Read the model definition and answer for the solid it produces. Units are mm, in the model's axes. Face numbers are marked on the shaded views. Coordinates: 2 decimals unless noted, no trailing zeros. Loops run counter-clockwise (first coordinate to the right, second up) from the corner with the lowest first, then second, coordinate; pieces in that order, holes last. Notation, with made-up numbers: (0, 72) - (11, 72) arc R22 cw to (11, 111) - close; hole circle Ø1 at (-30.5, 40.5). An arc over 180 degrees is marked (long way). Use CSV: the item, a comma, the result in double quotes.
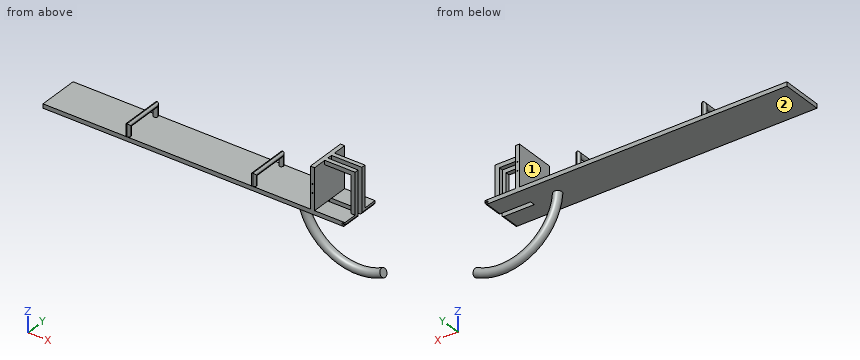
```python
from build123d import *

# Parameters (mm, degrees)
F1_DEPTH  = 20
F2_R      = 10
F5_R      = 20
F9_DEPTH  = 196.2
F11_R     = 2.5
F12_DEPTH = 30
F14_R     = 2.5
F15_DEPTH = 30
F18_DEPTH = 20
F21_DEPTH = 20
F23_DEPTH = 20
F26_DEPTH = 20


with BuildPart() as f1:
    # F0 (on Top) → F1 (new body)
    with BuildSketch(Plane.XY):
        Polygon((0, -98.1), (0, -12), (-155, -12), (-155, 0), (-155, 12), (0, 12), (0, 98.1), (-1441.76, 98.1), (-1441.76, -98.1), align=None)
    extrude(amount=-F1_DEPTH)

    # F2
    f2_edges = [f1.edges().sort_by_distance(p)[0] for p in [
        (0, -55.05, -20),
        (0, 55.05, -20),
    ]]
    fillet(f2_edges, radius=F2_R)

    # F6: sweep along a path in F4
    with BuildLine(Plane.XZ) as f6_path:
        ThreePointArc((-276.33, 0), (-148.7703707389, -227.3201555186), (111.7183092779, -236.8888390924))
    # F5 (on Top) → F6 (sweep)
    with BuildSketch(Plane.XY):
        with Locations((-276.33, 0)):
            Circle(F5_R)
    sweep(path=f6_path.line)

    # F8 (on offset) → F9 (join)
    with BuildSketch(Plane.XZ.offset(98.1)):
        Polygon((-155, 0), (-145, 0), (-145, 196.2), (-155, 196.2), (-165, 196.2), (-165, 0), align=None)
    extrude(amount=-F9_DEPTH)

    # F11 (on offset) → F12 (cut)
    with BuildSketch(Plane.XZ.offset(98.1)):
        with Locations((-155, 118.6)):
            Circle(F11_R)
        with Locations((-155, 77.6)):
            Circle(F11_R)
    extrude(amount=-F12_DEPTH, mode=Mode.SUBTRACT)

    # F14 (on offset) → F15 (cut)
    with BuildSketch(Plane(origin=(0, 98.1, 0), x_dir=(-1, 0, 0), z_dir=(0, 1, 0))):
        with Locations((155, 118.6)):
            Circle(F14_R)
        with Locations((155, 77.6)):
            Circle(F14_R)
    extrude(amount=-F15_DEPTH, mode=Mode.SUBTRACT)

    # F17 (on offset) → F18 (join)
    with BuildSketch(Plane.XZ.offset(-12)):
        Polygon((-20, 0), (0, 0), (0, 196.2), (-145, 196.2), (-145, 176.2), (-20, 176.2), align=None)
    extrude(amount=-F18_DEPTH)

    # F20 (on offset) → F21 (join)
    with BuildSketch(Plane(origin=(0, -12, 0), x_dir=(-1, 0, 0), z_dir=(0, 1, 0))):
        Polygon((0, 196.2), (0, 0), (20, 0), (20, 176.2), (145, 176.2), (145, 196.2), align=None)
    extrude(amount=-F21_DEPTH)

    # F22 (on offset) → F23 (cut)
    with BuildSketch(Plane.XZ.offset(98.1)):
        with BuildLine():
            ThreePointArc((-10, -5), (-13.5355339059, -13.5355339059), (-5, -10))
            ThreePointArc((-5, -10), (-6.4644660941, -6.4644660941), (-10, -5))
        make_face()
    extrude(amount=-F23_DEPTH, mode=Mode.SUBTRACT)

    # F25 (on offset) → F26 (cut)
    with BuildSketch(Plane(origin=(0, 98.1, 0), x_dir=(-1, 0, 0), z_dir=(0, 1, 0))):
        with BuildLine():
            ThreePointArc((10, -5), (6.4644660941, -13.5355339059), (15, -10))
            ThreePointArc((15, -10), (13.5355339059, -6.4644660941), (10, -5))
        make_face()
    extrude(amount=-F26_DEPTH, mode=Mode.SUBTRACT)

    # F29: sweep along a path in F28
    with BuildLine(Plane(origin=(-440, 0, 0), x_dir=(0, -1, 0), z_dir=(-1, 0, 0))) as f29_path:
        Line((88.1, 0), (88.1, 50))
        Line((88.1, 50), (-88.1, 50))
        Line((-88.1, 50), (-88.1, 0))
    # F3 (on Top) → F29 (sweep)
    with BuildSketch(Plane.XY):
        with BuildLine():
            ThreePointArc((-440, -98.1), (-432.9289321881, -95.1710678119), (-430, -88.1))
            ThreePointArc((-430, -88.1), (-447.0710678119, -81.0289321881), (-440, -98.1))
        make_face()
    sweep(path=f29_path.line, transition=Transition.RIGHT)

    # F32: sweep along a path in F31
    with BuildLine(Plane(origin=(-1040, 0, 0), x_dir=(0, -1, 0), z_dir=(-1, 0, 0))) as f32_path:
        Line((88.1, 0), (88.1, 50))
        Line((88.1, 50), (-88.1, 50))
        Line((-88.1, 50), (-88.1, 0))
    # F3 (on Top) → F32 (sweep)
    with BuildSketch(Plane.XY):
        with BuildLine():
            ThreePointArc((-1040, -98.1), (-1032.9289321881, -95.1710678119), (-1030, -88.1))
            ThreePointArc((-1030, -88.1), (-1047.0710678119, -81.0289321881), (-1040, -98.1))
        make_face()
    sweep(path=f32_path.line, transition=Transition.RIGHT)


solid = f1.part
```
Q1. For a pull along X with two mould halves and no side action, classify the marked faces 1 and 2 as +X half, -X half, draft (parallel to the pull), parting line (faces both ways), or undercut.
Reported:
face 1,"undercut"
face 2,"draft"
Q2. The part is cut by section A-A on x = -1073. Determine the outline of the cut face in (y, z), and give its area (3 significant figures).
Reported:
outline,"(-98.1, -20) - (98.1, -20) - (98.1, 0) - (-98.1, 0) - close"
area,"3,920 mm²"
Q3. Given P1, Ø6, axis at x = -183.5, y = -42, coming from the -Z side; P2, Ø10, axis at x = -95.5, y = 17, coming from the -Z side; P3, Ø22, axis at x = -89.5, y = -24.5, coming from the -Z side, each flat-ended and moving along its own axis, determine where each tip first touches the part or whether it passes through.
Reported:
P1,"stops at z = -20"
P2,"stops at z = -269.37"
P3,"stops at z = -270.07"
Q4. Find the intervals of material crossed by probe 1 along Z at (x, y) = (-155, 86.5); probe 2 along Z at (x, y) = (-77.5, 31); probe 3 along X at (y, z) = (-90, 77), in increasing order. Write a range as [from, to].
Reported:
probe 1,"z = [-20, 75.1], [80.1, 116.1], [121.1, 196.2]"
probe 2,"z = [-20, 0], [176.2, 196.2]"
probe 3,"x = [-165, -157.43], [-152.57, -145]"
